Job drawing, mm, ordinate dimensions from the low corner. One solid piece. A direction names the side the tool comes from. Coordinates: 2 decimals unless noted, no trailing zeros. Loops run counter-clockwise (first coordinate to the right, second up) from the corner with the lowest first, then second, coordinate; pieces in that order, holes last. Notation, with made-up numbers: M -15,20 L -6,20 A12 cw -6,30 Z; hole C -24,-16.75 d1. An arc over 180 degrees is marked long. Write each question's results on one line, items separated by ' | '. Start each with the question number.
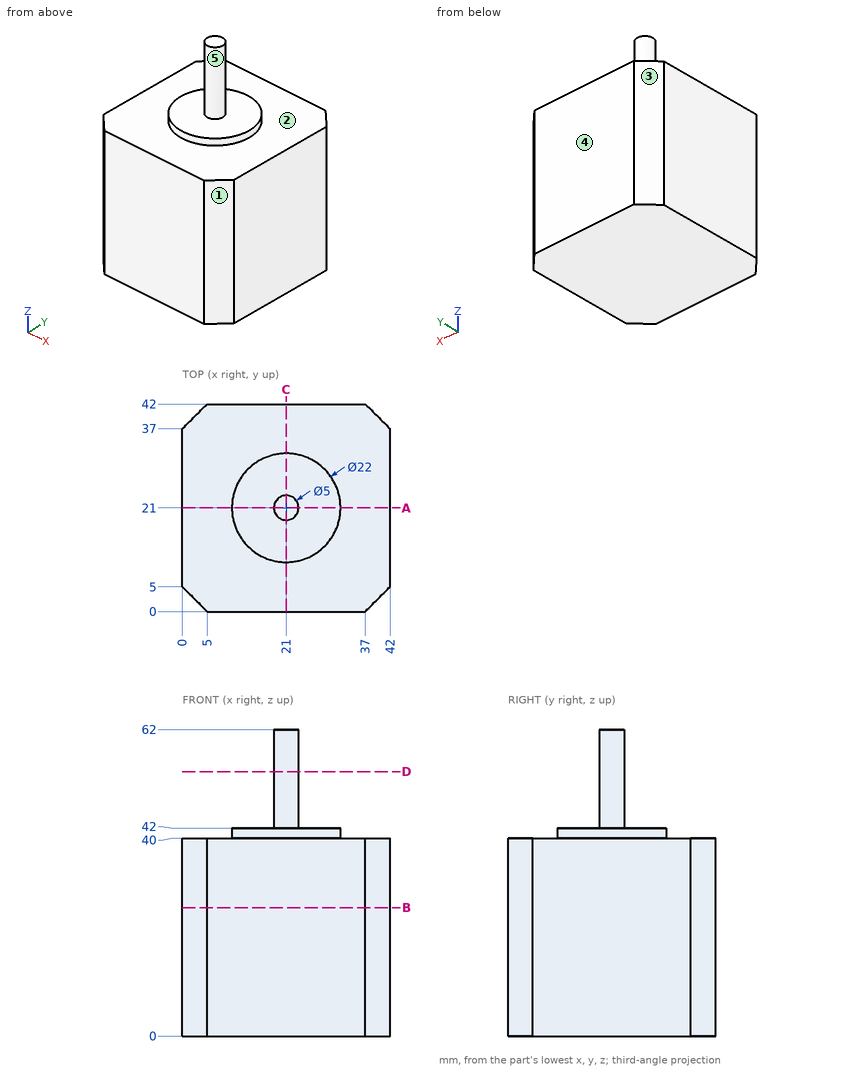
1. Band-saw the part on B-B, the plane z = 26. List the corners of the cut face in (x, y).
2. Band-saw the part on A-A, the plane y = 21. List the corners of the cut face in (x, z), plus the area to 3 significant figures.
3. Band-saw the part on D-D, the plane z = 53.5. List the corners of the cut face in (x, y).
4. Which spindle directions (+Z, -Z, +X, -X, +Y, -Y) get a long thin tool onto all of the face, cutting with end or side? Do the marked faces 4 and 5. Say none if no direction does.
5. Mould opens along X. For the marked faces 1, 2 and 3 say: +X half, -X half, draft (parallel to the pull), parting line (faces both ways), or undercut.
6. Wall check: line 1 along Z through (x, y) = (8, 14); line 2 along Z through (x, y) = (29, 20.5); line 3 along X through (y, z) = (38, 3). Give the ranges that are in metal, low to high.
7. Pin check, flat tip, straight feed: pin 1 (3 mm diameter, centred on y = 9, z = 34.5, fed in from -X). Stop position of the tip, or through.
Checked values:
1) outline: M 0,5 L 5,0 L 37,0 L 42,5 L 42,37 L 37,42 L 5,42 L 0,37 Z
2) outline: M 0,0 L 42,0 L 42,40 L 32,40 L 32,42 L 23.5,42 L 23.5,62 L 18.5,62 L 18.5,42 L 10,42 L 10,40 L 0,40 Z | area: 1,820 mm²
3) outline: C 21,21 d5
4) face 4: +Z, -Z, +X, -X, +Y | face 5: +Z
5) face 1: +X half | face 2: draft | face 3: -X half
6) line 1: 0 to 40 | line 2: 0 to 42 | line 3: 1 to 41
7) pin 1: x = 0
